Could you check a few things on this model? Use its own coordinates, in mm. Face numbers are marked on the shaded views. A direction names the side the tool comes from. Give positions to 0.01 mm unless a question says otherwise; leave off trailing zeros. Loops run counter-clockwise (first coordinate to the right, second up) from the corner with the lowest first, then second, coordinate; pieces in that order, holes last. Notation, with made-up numbers: (84, 50) -> (92, 50) arc R23 cw to (92, 60) -> close; hole circle Ø6 at (-16.5, -36). An arc over 180 degrees is marked (long way). Write each question's results on one line, items separated by ' | '. Start each with the question number.
Q1. Will these pins go through, and if not, where does the flat tip stop? P1, Ø1.5, axis at y = 85.5, z = 22.5, coming from the -X side; P2, Ø16.5, axis at x = -29.5, y = 83, coming from the -Z side; P3, Ø2, axis at y = 105.5, z = -14, coming from the +X side; P4, Ø4.5, axis at x = -1, y = 155, coming from the -Z side.
Q2. If we section it at A-A, the plane y = 135: List the corners of the cut face in (x, z) for me, plus the area to 3 significant figures.
Q3. Which directions (+Z, -Z, +X, -X, +Y, -Y) give clear straight access to the entire face, cutting with the end or side of a thin tool? Please do the marked faces 1 and 2.
Q4. If I drill on line 1 along X through (y, z) = (21, 24.5); line 2 along Z through (x, y) = (23.5, 10), over which ranges is the centre line in solid material (lowest first)?
Autodesk Inventor part; units mm, degrees
ref_plane "YZ Plane" through (0, 0, 0) normal (1, 0, 0) x (0, 1, 0)
ref_plane "XZ Plane" through (0, 0, 0) normal (0, 1, 0) x (-1, 0, 0)
ref_plane "XY Plane" through (0, 0, 0) normal (0, 0, 1) x (1, 0, 0)
sketch "Sketch1" plane through (0, 0, 0) normal (0, 1, 0) x (-1, 0, 0)
  line L0 (62.25, -32.4) -> (-62.25, -32.4)
  line L1 (-62.25, -32.4) -> (-62.25, 32.4)
  line L2 (-62.25, 32.4) -> (62.25, 32.4)
  line L3 (62.25, 32.4) -> (62.25, -32.4)
  point P0 (0, 0)
  point P1 (62.25, 0)
  point P2 (0, -32.4)
  dimension "d0" = 124.5
  dimension "d2" = 64.8
extrude "Extrusion1" add sketch "Sketch1" along normal blind 161
sketch "Sketch2" plane through (-62.25, 0, 32.4) normal (0, 0, 1) x (1, 0, 0)
  line L0 (124.5, 0) -> (0, 0)
  line L1 (124.5, 0) -> (124.5, 161)
  line L2 (0, 0) -> (0, 161)
  line L3 (0, 23) -> (124.5, 23)
  line L4 (124.5, 23) -> (124.5, 8)
  line L5 (124.5, 8) -> (0, 8)
  line L6 (0, 8) -> (0, 23)
  line L7 (0, 31) -> (124.5, 31)
  line L8 (124.5, 31) -> (124.5, 46)
  line L9 (124.5, 46) -> (0, 46)
  line L10 (0, 46) -> (0, 31)
  line L11 (0, 54) -> (124.5, 54)
  line L12 (124.5, 54) -> (124.5, 69)
  line L13 (124.5, 69) -> (0, 69)
  line L14 (0, 69) -> (0, 54)
  line L15 (0, 77) -> (124.5, 77)
  line L16 (124.5, 77) -> (124.5, 92)
  line L17 (124.5, 92) -> (0, 92)
  line L18 (0, 92) -> (0, 77)
  line L19 (0, 100) -> (124.5, 100)
  line L20 (124.5, 100) -> (124.5, 115)
  line L21 (124.5, 115) -> (0, 115)
  line L22 (0, 115) -> (0, 100)
  line L23 (0, 123) -> (124.5, 123)
  line L24 (124.5, 123) -> (124.5, 138)
  line L25 (124.5, 138) -> (0, 138)
  line L26 (0, 138) -> (0, 123)
  line L27 (124.5, 146) -> (0, 146)
  line L28 (0, 146) -> (0, 161)
  line L29 (0, 161) -> (124.5, 161)
  line L30 (124.5, 161) -> (124.5, 146)
  point P0 (62.25, 0)
  dimension "d5" = 8
  dimension "d6" = 15
  dimension "d7" = 8
  dimension "d8" = 15
  dimension "d9" = 8
  dimension "d10" = 15
  dimension "d11" = 8
  dimension "d12" = 15
  dimension "d13" = 8
  dimension "d14" = 8
  dimension "d15" = 15
  dimension "d16" = 15
  dimension "d17" = 8
  dimension "d18" = 15
sketch "Sketch3" plane through (62.25, 0, -32.4) normal (0, 0, -1) x (-1, 0, 0)
  line L0 (0, 161) -> (124.5, 161)
  line L1 (0, 23) -> (124.5, 23)
  line L2 (124.5, 23) -> (124.5, 8)
  line L3 (124.5, 8) -> (0, 8)
  line L4 (0, 8) -> (0, 23)
  line L5 (0, 31) -> (124.5, 31)
  line L6 (124.5, 31) -> (124.5, 46)
  line L7 (124.5, 46) -> (0, 46)
  line L8 (0, 46) -> (0, 31)
  line L9 (0, 54) -> (124.5, 54)
  line L10 (124.5, 54) -> (124.5, 69)
  line L11 (124.5, 69) -> (0, 69)
  line L12 (0, 69) -> (0, 54)
  line L13 (0, 77) -> (124.5, 77)
  line L14 (124.5, 77) -> (124.5, 92)
  line L15 (124.5, 92) -> (0, 92)
  line L16 (0, 92) -> (0, 77)
  line L17 (0, 100) -> (124.5, 100)
  line L18 (124.5, 100) -> (124.5, 115)
  line L19 (124.5, 115) -> (0, 115)
  line L20 (0, 115) -> (0, 100)
  line L21 (0, 123) -> (124.5, 123)
  line L22 (124.5, 123) -> (124.5, 138)
  line L23 (124.5, 138) -> (0, 138)
  line L24 (0, 138) -> (0, 123)
  line L25 (124.5, 146) -> (0, 146)
  line L26 (0, 146) -> (0, 161)
  line L27 (0, 161) -> (124.5, 161)
  line L28 (124.5, 161) -> (124.5, 146)
  point P0 (62.25, 0)
  point P1 (62.25, 0)
  dimension "d20" = 15
  dimension "d21" = 8
  dimension "d22" = 15
  dimension "d23" = 8
  dimension "d24" = 15
  dimension "d25" = 8
  dimension "d26" = 15
  dimension "d27" = 8
  dimension "d28" = 8
  dimension "d29" = 15
  dimension "d30" = 15
  dimension "d31" = 8
  dimension "d32" = 15
extrude "Extrusion2" cut sketch "Sketch3" against normal blind 1.5
extrude "Extrusion3" cut sketch "Sketch2" against normal blind 1.5 contours L5 L2 L3 L1 | L7 L2 L9 L1 | L11 L2 L13 L1 | L15 L2 L17 L1 | L19 L2 L21 L1 | L23 L2 L25 L1 | L27 L2 L29 L1
sketch "Sketch5" plane through (62.25, 0, 32.4) normal (1, 0, 0) x (0, 0, -1)
  line L0 (1.5, 161) -> (63.3, 161)
  line L1 (63.3, 161) -> (63.3, 146)
  line L2 (63.3, 146) -> (1.5, 146)
  line L3 (1.5, 146) -> (1.5, 161)
  line L4 (1.5, 138) -> (63.3, 138)
  line L5 (63.3, 138) -> (63.3, 123)
  line L6 (63.3, 123) -> (1.5, 123)
  line L7 (1.5, 123) -> (1.5, 138)
  line L8 (1.5, 115) -> (63.3, 115)
  line L9 (63.3, 115) -> (63.3, 100)
  line L10 (63.3, 100) -> (1.5, 100)
  line L11 (1.5, 100) -> (1.5, 115)
  line L12 (1.5, 92) -> (63.3, 92)
  line L13 (63.3, 92) -> (63.3, 77)
  line L14 (63.3, 77) -> (1.5, 77)
  line L15 (1.5, 77) -> (1.5, 92)
  line L16 (1.5, 69) -> (63.3, 69)
  line L17 (63.3, 69) -> (63.3, 54)
  line L18 (63.3, 54) -> (1.5, 54)
  line L19 (1.5, 54) -> (1.5, 69)
  line L20 (1.5, 46) -> (63.3, 46)
  line L21 (63.3, 46) -> (63.3, 31)
  line L22 (63.3, 31) -> (1.5, 31)
  line L23 (1.5, 31) -> (1.5, 46)
  line L24 (1.5, 23) -> (63.3, 23)
  line L25 (63.3, 23) -> (63.3, 8)
  line L26 (63.3, 8) -> (1.5, 8)
  line L27 (1.5, 8) -> (1.5, 23)
  point P0 (32.4, 0)
sketch "Sketch6" plane through (-62.25, 0, -32.4) normal (-1, 0, 0) x (0, 0, 1)
  line L0 (1.5, 161) -> (63.3, 161)
  line L1 (1.5, 161) -> (1.5, 146)
  line L2 (1.5, 161) -> (63.3, 161)
  line L3 (63.3, 161) -> (63.3, 146)
  line L4 (63.3, 146) -> (1.5, 146)
  line L5 (1.5, 146) -> (1.5, 161)
  line L6 (63.3, 138) -> (1.5, 138)
  line L7 (1.5, 138) -> (1.5, 123)
  line L8 (1.5, 123) -> (63.3, 123)
  line L9 (63.3, 123) -> (63.3, 138)
  line L10 (1.5, 115) -> (63.3, 115)
  line L11 (63.3, 115) -> (63.3, 100)
  line L12 (63.3, 100) -> (1.5, 100)
  line L13 (1.5, 100) -> (1.5, 115)
  line L14 (1.5, 92) -> (63.3, 92)
  line L15 (63.3, 92) -> (63.3, 77)
  line L16 (63.3, 77) -> (1.5, 77)
  line L17 (1.5, 77) -> (1.5, 92)
  line L18 (63.3, 69) -> (1.5, 69)
  line L19 (1.5, 69) -> (1.5, 54)
  line L20 (1.5, 54) -> (63.3, 54)
  line L21 (63.3, 54) -> (63.3, 69)
  line L22 (1.5, 46) -> (63.3, 46)
  line L23 (63.3, 46) -> (63.3, 31)
  line L24 (63.3, 31) -> (1.5, 31)
  line L25 (1.5, 31) -> (1.5, 46)
  line L26 (63.3, 23) -> (1.5, 23)
  line L27 (1.5, 23) -> (1.5, 8)
  line L28 (1.5, 8) -> (63.3, 8)
  line L29 (63.3, 8) -> (63.3, 23)
  point P0 (32.4, 0)
extrude "Extrusion4" cut sketch "Sketch6" against normal blind 1.5
extrude "Extrusion5" cut sketch "Sketch5" against normal blind 1.5
equation "\"d0\" = BtWd"
equation "\"d2\" = BtDp"
equation "\"d3\" = BatteryHt"
equation "\"d5\" = RidgeWd"
equation "\"d6\" = RidgeGapWd"
equation "\"d7\" = d5"
equation "\"d8\" = d6"
equation "\"d9\" = d7"
equation "\"d10\" = d6"
equation "\"d11\" = d5"
equation "\"d12\" = d6"
equation "\"d13\" = d5"
equation "\"d14\" = d5"
equation "\"d15\" = d6"
equation "\"d16\" = d15"
equation "\"d17\" = d14"
equation "\"d18\" = d16"
equation "\"d20\" = d34"
equation "\"d21\" = d19"
equation "\"d22\" = d20"
equation "\"d23\" = d21"
equation "\"d24\" = d20"
equation "\"d25\" = d19"
equation "\"d26\" = d20"
equation "\"d27\" = d19"
equation "\"d28\" = d19"
equation "\"d29\" = d20"
equation "\"d30\" = d29"
equation "\"d31\" = d28"
equation "\"d32\" = d30"
equation "\"d36\" = RidgeThickness"
equation "\"d38\" = RidgeThickness"
equation "\"d40\" = RidgeThickness"
equation "\"d42\" = RidgeThickness"
equation "\"d19\" = d33"
properties part number "L16-TSV-8.1"
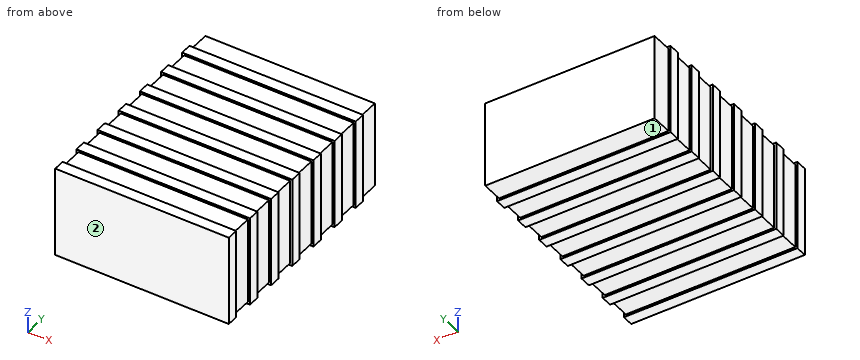
Final values:
1) P1: stops at x = -60.75 | P2: stops at z = -32.4 | P3: stops at x = 60.75 | P4: stops at z = -30.9
2) outline: (-60.75, -30.9) -> (60.75, -30.9) -> (60.75, 30.9) -> (-60.75, 30.9) -> close | area: 7,510 mm²
3) face 1: -Z, +X, -X, +Y | face 2: +Z, -Z, +X, -X, -Y
4) line 1: x = -60.75 to 60.75 | line 2: z = -30.9 to 30.9
